from build123d import *

# Parameters (mm, degrees)
PAD_DEPTH = 1


with BuildPart() as part:
    # Sketch → Pad (new body)
    with BuildSketch(Plane.YZ.offset(-500)):
        with BuildLine():
            ThreePointArc((-427.08313, 260), (-498.445232, -39.399887), (-380.9308, -323.869921))
            Line((-380.9308, -323.869921), (-600, -507.690796))
            Line((-600, -507.690796), (-600, -1400))
            Line((-600, -1400), (600, -1400))
            Line((600, -1400), (600, -507.690796))
            Line((600, -507.690796), (380.9308, -323.869921))
            ThreePointArc((380.9308, -323.869921), (465.068634, -183.606008), (499.438281, -23.693945))
            Line((499.438281, 340), (499.438281, -23.693945))
            Line((380, 340), (499.438281, 340))
            Line((380, 460), (380, 340))
            Line((230, 460), (380, 460))
            Line((230, 530), (230, 460))
            Line((0, 530), (230, 530))
            Line((0, 1040), (0, 530))
            Line((-658.874021, 1040), (0, 1040))
            Line((-658.874021, 1040), (-658.874021, 540))
            Line((-427.08313, 260), (-658.874021, 540))
        make_face()
    extrude(amount=-PAD_DEPTH)


solid = part.part
Check sheet for the modelled part. Datum: model origin and axes. Units: mm. A direction names the side the tool comes from. Give positions to 0.01 mm unless a question says otherwise; leave off trailing zeros. Write each loop counter-clockwise with the first axis right and the second up, starting at its lowest first coordinate (ties: lowest second). Pieces come first, ordered by that corner, then holes. Notation, with made-up numbers: (77.25, 7.25) -> (84.25, 7.25) arc R19 ccw to (84.25, 30.25) -> close; hole circle Ø4 at (-14, 68). An arc over 180 degrees is marked (long way). Use one line per item in the form item = value. Start each with the question number.
1. Access from +Z, -Z, +X, -X, +Y, -Y to the whole of each face (thin tool, end or side, straight path). Record for faces 1 (the flat face through (-500, -38, -434)), 2 (the flat face through (-500.49, -488.93, -414.49)), 3 (the cylindrical face through (-500.49, 464.22, -185.74)).
2. Section check C-C (z = -938.5). Record the cut outline in (x, y).
3. Mould release check, pull along Z, two halves, no side actions. Record for faces 4 (the flat face through (-500.49, 492, -417.07)), 5 (the flat face through (-501, -38, -434)), 6 (the cylindrical face through (-500.49, -498.77, -35.03)): pulls with the +Z half, pulls with the -Z half, needs draft (parallel to the pull), parting line crosses it, or undercut.
4. Section check B-B (x = -500.45). Record the cut outline in (y, z).
5. Section check A-A (y = 405.5). Record the cut outline in (x, z), and give its area (3 significant figures).
6. Thickness scan on line 1 along Z through (x, y) = (-500.3, 1); line 2 along Z through (x, y) = (-500.45, 287); line 3 along Y through (x, z) = (-500.35, 692.5). Record the ranges inside material, lowest first. Write a range as from..to.
7. Go/stop test with flat-tipped pins: P1, Ø0.5, axis at x = -500.5, y = 435.5, coming from the +Z side; P2, Ø0.5, axis at x = -500.5, z = 672.5, coming from the +Y side. Record where each tip stops, or that it passes through.
8. Section check D-D (y = 84). Record the cut outline in (x, z), and give its area (3 significant figures).
Conclusion:
q1.face_1 = +Z, -Z, +X, +Y, -Y
q1.face_2 = +X, -X, -Y
q1.face_3 = +X, -X, +Y
q2.outline = (-501, -600) -> (-500, -600) -> (-500, 600) -> (-501, 600) -> close
q3.face_4 = undercut
q3.face_5 = needs draft
q3.face_6 = undercut
q4.outline = (-658.87, 540) -> (-427.08, 260) arc R500 ccw to (-380.93, -323.87) -> (-600, -507.69) -> (-600, -1400) -> (600, -1400) -> (600, -507.69) -> (380.93, -323.87) arc R500 ccw to (499.44, -23.69) -> (499.44, 340) -> (380, 340) -> (380, 460) -> (230, 460) -> (230, 530) -> (0, 530) -> (0, 1040) -> (-658.87, 1040) -> close
q5.outline = (-501, -1400) -> (-500, -1400) -> (-500, -344.49) -> (-501, -344.49) -> close; (-501, -292.52) -> (-500, -292.52) -> (-500, 340) -> (-501, 340) -> close
q5.area = 1,690 mm²
q6.line_1 = -1400..530
q6.line_2 = -1400..460
q6.line_3 = -658.87..0
q7.P1 = 340
q7.P2 = 0
q8.outline = (-501, -1400) -> (-500, -1400) -> (-500, 530) -> (-501, 530) -> close
q8.area = 1,930 mm²
